Check sheet for the modelled part. Datum: model origin and axes. Units: mm. Give positions to 0.01 mm unless a question says otherwise; leave off trailing zeros.
from build123d import *

# Parameters (mm, degrees)
SKETCH1_W           = 150
SKETCH1_H           = 40
BOSS_EXTRUDE1_DEPTH = 2
SKETCH2_R           = 1.75
CUT_EXTRUDE1_DEPTH  = 3
FILLET1_R           = 5


with BuildPart() as part:
    # Sketch1 → Boss-Extrude1 (new body)
    with BuildSketch(Plane.XY):
        Rectangle(SKETCH1_W, SKETCH1_H)
    extrude(amount=BOSS_EXTRUDE1_DEPTH)

    # Sketch2 → Cut-Extrude1 (cut, through all)
    with BuildSketch(Plane.XY.offset(2)):
        with Locations((-70, 15)):
            Circle(SKETCH2_R)
        with Locations((-70, -15)):
            Circle(SKETCH2_R)
        with Locations((70, -15)):
            Circle(SKETCH2_R)
        with Locations((70, 15)):
            Circle(SKETCH2_R)
    extrude(amount=-CUT_EXTRUDE1_DEPTH, mode=Mode.SUBTRACT)

    # Fillet1
    fillet1_edges = [part.edges().sort_by_distance(p)[0] for p in [
        (-75, 20, 1),
        (75, 20, 1),
        (75, -20, 1),
        (-75, -20, 1),
    ]]
    fillet(fillet1_edges, radius=FILLET1_R)


solid = part.part
1) Draft check along Y on faces 1 (the face through (-1, 0, 2)), 2 (the face through (-68.331, 15.526, 1.014)), 3 (the face through (73, 19, 1)), 4 (the face through (73, -19, 1)). Enter one of: +Y half, -Y half, draft (parallel to the pull), parting line (faces both ways), or undercut.
Recorded:
face 1: draft
face 2: undercut
face 3: +Y half
face 4: -Y half
2) Depth check by flat-ended pin: pin 1 Ø3 at (x, y) = (-70, -15) entering from -Z. Enter the tip coordinate at first touch or a pass-through.
Recorded:
pin 1: passes through
3) Material ranges on L1, parallel to Y at x = 70, z = 1.15; L2, parallel to X at y = -14, z = 1.4; L3, parallel to X at y = 14.5, z = 0.85, recorded low to high.
Recorded:
L1: y = -20 to -16.75, -13.25 to 13.25, 16.75 to 20
L2: x = -75 to -71.44, -68.56 to 68.56, 71.44 to 75
L3: x = -75 to -71.68, -68.32 to 68.32, 71.68 to 75
